```python
from build123d import *

# Parameters (mm, degrees)
SKETCH1_W               = 50
SKETCH1_H               = 10
BOSS_EXTRUDE1_DEPTH     = 5
CUT_EXTRUDE1_DEPTH      = 6
CUT_EXTRUDE1_DEPTH_BACK = 6
SKETCH3_W               = 45.6
SKETCH3_H               = 2.6
BOSS_EXTRUDE2_DEPTH     = 77
SKETCH4_W               = 39.8
SKETCH4_H               = 72
CUT_EXTRUDE2_DEPTH      = 77
BOSS_EXTRUDE3_DEPTH     = 72
SKETCH7_W               = 39.8
SKETCH7_H               = 3
CUT_EXTRUDE3_DEPTH      = 10


with BuildPart() as part:
    # Sketch1 → Boss-Extrude1 (new body)
    with BuildSketch(Plane.XY):
        Rectangle(SKETCH1_W, SKETCH1_H)
    extrude(amount=BOSS_EXTRUDE1_DEPTH)

    # Sketch2 → Cut-Extrude1 (cut, two sides)
    with BuildSketch(Plane(origin=(0, 0, 0), x_dir=(1, 0, 0), z_dir=(0, 1, 0))) as cut_extrude1_sk:
        Polygon((-25, -5), (-20, 0), (-25, 0), align=None)
        Polygon((25, -5), (20, 0), (25, 0), align=None)
    extrude(amount=CUT_EXTRUDE1_DEPTH, mode=Mode.SUBTRACT)
    extrude(cut_extrude1_sk.sketch, amount=-CUT_EXTRUDE1_DEPTH_BACK, mode=Mode.SUBTRACT)

    # Sketch3 → Boss-Extrude2 (add)
    with BuildSketch(Plane.XY.offset(5)):
        Rectangle(SKETCH3_W, SKETCH3_H)
    extrude(amount=-BOSS_EXTRUDE2_DEPTH)

    # Sketch4 → Cut-Extrude2 (cut)
    with BuildSketch(Plane(origin=(0, 1.3, 0), x_dir=(1, 0, 0), z_dir=(0, 1, 0))):
        with Locations((0, 36)):
            Rectangle(SKETCH4_W, SKETCH4_H)
    extrude(amount=-CUT_EXTRUDE2_DEPTH, mode=Mode.SUBTRACT)

    # Sketch6 → Boss-Extrude3 (add)
    with BuildSketch(Plane(origin=(0, 0, 0), x_dir=(-1, 0, 0), z_dir=(0, 0, -1))):
        Polygon((-19.9, -1.3), (-19.9, 5), (19.9, 5), (19.9, -1.3), (18.4, -1.3), (18.4, 3), (-18.4, 3), (-18.4, -1.3), align=None)
    extrude(amount=BOSS_EXTRUDE3_DEPTH)

    # Sketch7 → Cut-Extrude3 (cut)
    with BuildSketch(Plane(origin=(0, 5, 0), x_dir=(1, 0, 0), z_dir=(0, 1, 0))):
        with Locations((0, 70.5)):
            Rectangle(SKETCH7_W, SKETCH7_H)
    extrude(amount=-CUT_EXTRUDE3_DEPTH, mode=Mode.SUBTRACT)


solid = part.part
```
The model under review builds one solid part; all positions refer to its coordinate system, in mm. A direction names the side the tool comes from. Give positions to 0.01 mm unless a question says otherwise; leave off trailing zeros. Write each loop counter-clockwise with the first axis right and the second up, starting at its lowest first coordinate (ties: lowest second). Pieces come first, ordered by that corner, then holes. Notation, with made-up numbers: M -32.75,87.5 L 21.25,87.5 A20 cw 21.25,113.5 Z; hole C 70,63 d5. An arc over 180 degrees is marked long. Write each question's results on one line, items separated by ' | '. Start each with the question number.
1. We need section D-D (y = -3). Write out the cut boundary in (x, z).
2. Insertion check: pin 1 Ø3 at (x, y) = (17, -1) entering from -Z; pin 2 Ø1.3 at (y, z) = (0.5, -44.5) entering from -X; pin 3 Ø1.5 at (x, y) = (-8, 0.5) entering from -Z. Each pin has a flat end and moves straight along its axis. Give the tip position at first contact, or say it passes through.
3. Mouldability with a two-part tool opening along X and no side actions: class faces 1 (the flat face through (-19.9, 3, -34)), 2 (the flat face through (-18.4, 1, -34)), 3 (the flat face through (-21, 0, -72)) as released by +X, released by -X, zero draft, split by the parting line, or undercut.
4. We need section A-A (z = -28). Write out the cut boundary in (x, y).
5. We need section C-C (x = -9). Write out the cut boundary in (y, z).
6. For faces 4 (the flat face through (18.4, 1, -34)), 5 (the flat face through (-19.9, 0, -70)), 6 (the flat face through (19.9, 3, -34)), list the 3-axis set-ups (+Z, -Z, +X, -X, +Y, -Y) from which the entire face can be reached by the end or side of a thin tool; tool diameter is ignored.
7. We need section B-B (y = 4.25). Write out the cut boundary in (x, z).
8. For probe 1 along X at (y, z) = (0.5, -22); probe 2 along X at (y, z) = (2.5, -48.5); probe 3 along Y at (x, z) = (-9, -58.5), list the stretches that pass through material, from the lowest coordinate up. Write a range as [from, to].
Results found:
1) outline: M -25,5 L -20,0 L 20,0 L 25,5 Z
2) pin 1: stops at z = -69 | pin 2: stops at x = -22.8 | pin 3: stops at z = 0
3) face 1: released by -X | face 2: undercut | face 3: zero draft
4) outline: M -22.8,-1.3 L -18.4,-1.3 L -18.4,3 L 18.4,3 L 18.4,-1.3 L 22.8,-1.3 L 22.8,1.3 L 19.9,1.3 L 19.9,5 L -19.9,5 L -19.9,1.3 L -22.8,1.3 Z
5) outline: M -5,0 L 3,0 L 3,-69 L 5,-69 L 5,5 L -5,5 Z
6) face 4: -Z, -Y | face 5: -Z, +Y, -Y | face 6: -Z, +X, +Y
7) outline: M -25,5 L -20,0 L -19.9,0 L -19.9,-69 L 19.9,-69 L 19.9,0 L 20,0 L 25,5 Z
8) probe 1: x = [-22.8, -18.4], [18.4, 22.8] | probe 2: x = [-19.9, -18.4], [18.4, 19.9] | probe 3: y = [3, 5]
